```python
from build123d import *

# Parameters (mm, degrees)
CROQUIS1_W              = 46
CROQUIS1_H              = 42
SALIENTE_EXTRUIR1_DEPTH = 4
CROQUIS3_W              = 2
CROQUIS3_H              = 42
SALIENTE_EXTRUIR2_DEPTH = 46
CROQUIS4_W              = 2
CROQUIS4_H              = 42
SALIENTE_EXTRUIR3_DEPTH = 15
CROQUIS6_W              = 2
CROQUIS6_H              = 42
SALIENTE_EXTRUIR4_DEPTH = 15
CROQUIS8_R              = 1.25
CORTAR_EXTRUIR1_DEPTH   = 15
CORTAR_EXTRUIR2_DEPTH   = 15
CROQUIS10_R             = 1.25
CORTAR_EXTRUIR4_DEPTH   = 15
REDONDEO1_R             = 3
REDONDEO2_R             = 3
CROQUIS11_R             = 10
CORTAR_EXTRUIR5_DEPTH   = 15


with BuildPart() as part:
    # Croquis1 → Saliente-Extruir1 (new body)
    with BuildSketch(Plane.XY):
        with Locations((-61.749794594, 15.620374367)):
            Rectangle(CROQUIS1_W, CROQUIS1_H)
    extrude(amount=SALIENTE_EXTRUIR1_DEPTH)

    # Croquis3 → Saliente-Extruir2 (add)
    with BuildSketch(Plane(origin=(0, 0, 0), x_dir=(-1, 0, 0), z_dir=(0, 0, -1))):
        with Locations((83.749794594, 15.620374367)):
            Rectangle(CROQUIS3_W, CROQUIS3_H)
        with Locations((39.749794594, 15.620374367)):
            Rectangle(CROQUIS3_W, CROQUIS3_H)
    extrude(amount=SALIENTE_EXTRUIR2_DEPTH)

    # Croquis4 → Saliente-Extruir3 (add)
    with BuildSketch(Plane.ZY.offset(84.749794594)):
        with Locations((-45, 15.620374367)):
            Rectangle(CROQUIS4_W, CROQUIS4_H)
    extrude(amount=SALIENTE_EXTRUIR3_DEPTH)

    # Croquis6 → Saliente-Extruir4 (add)
    with BuildSketch(Plane(origin=(-38.749794594, 0, 0), x_dir=(0, 0, -1), z_dir=(1, 0, 0))):
        with Locations((45, 15.620374367)):
            Rectangle(CROQUIS6_W, CROQUIS6_H)
    extrude(amount=SALIENTE_EXTRUIR4_DEPTH)

    # Croquis8 → Cortar-Extruir1 (cut)
    with BuildSketch(Plane.XY.offset(4)):
        with Locations((-45.499794594, 31.870374367)):
            Circle(CROQUIS8_R)
        with BuildLine():
            ThreePointArc((-79.249794594, -0.629625633), (-78.88367807, -1.51350911), (-77.999794594, -1.879625633))
            Line((-77.999794594, -1.879625633), (-77.999794594, -0.629625633))
            Line((-77.999794594, -0.629625633), (-79.249794594, -0.629625633))
        make_face()
        with BuildLine():
            Line((-77.999794594, -0.629625633), (-77.999794594, -1.879625633))
            ThreePointArc((-77.999794594, -1.879625633), (-77.115911117, -1.51350911), (-76.749794594, -0.629625633))
            ThreePointArc((-76.749794594, -0.629625633), (-77.999794594, 0.620374367), (-79.249794594, -0.629625633))
            Line((-79.249794594, -0.629625633), (-77.999794594, -0.629625633))
        make_face()
        with Locations((-77.999794594, 31.870374367)):
            Circle(CROQUIS8_R)
    extrude(amount=-CORTAR_EXTRUIR1_DEPTH, mode=Mode.SUBTRACT)

    # Croquis7 → Cortar-Extruir2 (cut)
    with BuildSketch(Plane.XY.offset(4)):
        with BuildLine():
            ThreePointArc((-44.249794594, -0.629625633), (-46.38367807, 0.254257843), (-45.499794594, -1.879625633))
            Line((-45.499794594, -1.879625633), (-45.499794594, -0.629625633))
            Line((-45.499794594, -0.629625633), (-44.249794594, -0.629625633))
        make_face()
        with BuildLine():
            Line((-45.499794594, -0.629625633), (-45.499794594, -1.879625633))
            ThreePointArc((-45.499794594, -1.879625633), (-44.615911117, -1.51350911), (-44.249794594, -0.629625633))
            Line((-44.249794594, -0.629625633), (-45.499794594, -0.629625633))
        make_face()
    extrude(amount=-CORTAR_EXTRUIR2_DEPTH, mode=Mode.SUBTRACT)

    # Croquis10 → Cortar-Extruir4 (cut)
    with BuildSketch(Plane.XY.offset(-44)):
        with Locations((-33.749794594, 31.620374367)):
            Circle(CROQUIS10_R)
        with Locations((-33.829898146, -0.379625633)):
            Circle(CROQUIS10_R)
    cortar_extruir4 = extrude(amount=-CORTAR_EXTRUIR4_DEPTH, mode=Mode.SUBTRACT)

    # Simetría1: Cortar-Extruir4 across plane
    add(cortar_extruir4.mirror(Plane(origin=(-61.749794594, 0, 0), x_dir=(0, 0, 1), z_dir=(1, 0, 0))), mode=Mode.SUBTRACT)

    # Redondeo1
    redondeo1_edges = [part.edges().sort_by_distance(p)[0] for p in [
        (-84.749794594, 15.620374367, -44),
    ]]
    fillet(redondeo1_edges, radius=REDONDEO1_R)

    # Redondeo2
    redondeo2_edges = [part.edges().sort_by_distance(p)[0] for p in [
        (-38.749794594, 15.620374367, -44),
    ]]
    fillet(redondeo2_edges, radius=REDONDEO2_R)

    # Croquis11 → Cortar-Extruir5 (cut)
    with BuildSketch(Plane.XY.offset(4)):
        with Locations((-61.749794594, 15.620374367)):
            Circle(CROQUIS11_R)
    extrude(amount=-CORTAR_EXTRUIR5_DEPTH, mode=Mode.SUBTRACT)


solid = part.part
```
The listing builds one solid part. Answer for the finished solid, in the listing's coordinates (mm). A direction names the side the tool comes from. Coordinates: 2 decimals unless noted, no trailing zeros. Order: outer loops, then holes, each group sorted by start corner. A loop starts at its lowest first (then second) coordinate and runs counter-clockwise, first axis right, second up. Notation, with made-up numbers: M -21,4 L 20,4 A18 ccw 20,36 Z; hole C 41.25,-14 d8. An arc over 180 degrees is marked long. Answer as a JSON object with one key per item and string values. Group by question number.
1. Determine the mould class of faces 1 (the cylindrical face through (-44.923, 30.761, 2.028)), 2 (the flat face through (-62, 36.62, 1)), 3 (the cylindrical face through (-85.65, 15.91, -43.14)) for opening direction Y: released by +Y, released by -Y, zero draft, split by the parting line, or undercut.
2. Section D-D on y = 4.5 is taken. Write down the section's boundary in (x, z).
3. Flat-ended cylindrical pins translate along their axes: P1, Ø12, axis at y = 14, z = -5.5, coming from the -X side; P2, Ø3, axis at x = -33.75, y = 31.62, coming from the +Z side; P3, Ø2, axis at y = 24.5, z = -9.5, coming from the +X side; P4, Ø10, axis at x = -49.5, z = -37, coming from the -Y side. Find the tip coordinate at first contact, or state that the pin passes through.
4. Straight lines are drawn through the part: line 1 (X direction, y = 24, z = -18); line 2 (Z direction, x = -36, y = -0.5); line 3 (Z direction, x = -69.5, y = 28.5). For each, find the intervals that lie inside material, in ascending order.
5. A tool of negligible diameter and unlimited length cuts with its end or side. For faces 4 (the flat face through (-32, 15, -46)), 5 (the flat face through (-84.75, 15, -18)), 6 (the flat face through (-53, 21, 0)), 7 (the flat face through (-38.75, 15, -19)), from which of +Z, -Z, +X, -X, +Y, -Y can it reach the whole face along a straight path? Write none if from no direction.
6. Section A-A on z = -22 is taken. Write down the section's boundary in (x, y), then the cut area to 3 significant figures.
7. Section C-C on x = -70.5 is taken. Write down the section's boundary in (y, z), then the cut area to 3 significant figures.
8. Section B-B on y = 12 is taken. Write down the section's boundary in (x, z).
Values follow:
{
 "1": {"face 1": "undercut", "face 2": "released by +Y", "face 3": "zero draft"},
 "2": {"outline": "M -99.75,-46 L -82.75,-46 L -82.75,0 L -40.75,0 L -40.75,-46 L -23.75,-46 L -23.75,-44 L -35.75,-44 A3 cw -38.75,-41 L -38.75,4 L -84.75,4 L -84.75,-41 A3 cw -87.75,-44 L -99.75,-44 Z"},
 "3": {"P1": "x = -84.75", "P2": "z = -44", "P3": "x = -38.75", "P4": "through"},
 "4": {"line 1": "-84.75 to -82.75, -40.75 to -38.75", "line 2": "-46 to -43.99", "line 3": "0 to 4"},
 "5": {"face 4": "-Z, +X, -X, +Y, -Y", "face 5": "+Z, -X, +Y, -Y", "face 6": "-Z, +Y, -Y", "face 7": "+Z, +X, +Y, -Y"},
 "6": {"outline": "M -84.75,-5.38 L -82.75,-5.38 L -82.75,36.62 L -84.75,36.62 Z; M -40.75,-5.38 L -38.75,-5.38 L -38.75,36.62 L -40.75,36.62 Z", "area": "168 mm2"},
 "7": {"outline": "M -5.38,0 L 10.78,0 L 10.78,4 L -5.38,4 Z; M 20.46,0 L 36.62,0 L 36.62,4 L 20.46,4 Z", "area": "129 mm2"},
 "8": {"outline": "M -99.75,-46 L -82.75,-46 L -82.75,0 L -71.07,0 L -71.07,4 L -84.75,4 L -84.75,-41 A3 cw -87.75,-44 L -99.75,-44 Z; M -52.43,0 L -40.75,0 L -40.75,-46 L -23.75,-46 L -23.75,-44 L -35.75,-44 A3 cw -38.75,-41 L -38.75,4 L -52.43,4 Z"}
}
